from build123d import *

# Parameters (mm, degrees)
SKETCH1_W                      = 80
SKETCH1_H                      = 342
BOSS_EXTRUDE1_DEPTH            = 18
FILLET1_R                      = 50
CBORE_FOR_M5_SHCS1_D           = 5.5
CBORE_FOR_M5_SHCS1_DEPTH       = 28.347633298
CBORE_FOR_M5_SHCS1_CBORE_D     = 10
CBORE_FOR_M5_SHCS1_CBORE_DEPTH = 5
CBORE_FOR_M5_SHCS1_TIP         = 1.652366702
CHAMFER1_SIZE                  = 1
SKETCH5_R                      = 3.25
CUT_EXTRUDE1_DEPTH             = 284.418418597
CHAMFER2_SIZE                  = 1


with BuildPart() as part:
    # Sketch1 → Boss-Extrude1 (new body)
    with BuildSketch(Plane.XY):
        with Locations((41, 100)):
            Rectangle(SKETCH1_W, SKETCH1_H)
    extrude(amount=BOSS_EXTRUDE1_DEPTH)

    # Fillet1
    fillet1_edges = [part.edges().sort_by_distance(p)[0] for p in [
        (81, 271, 9),
        (81, -71, 9),
    ]]
    fillet(fillet1_edges, radius=FILLET1_R)

    # CBORE for M5 SHCS1
    with Locations(Plane.XY.offset(18)):
        with Locations((9.25, 250), (9.25, 190), (9.25, 130), (9.25, 70), (9.25, 10), (9.25, -50)):
            CounterBoreHole(CBORE_FOR_M5_SHCS1_D / 2, CBORE_FOR_M5_SHCS1_CBORE_D / 2, CBORE_FOR_M5_SHCS1_CBORE_DEPTH, depth=CBORE_FOR_M5_SHCS1_DEPTH)
            with Locations((0, 0, -(CBORE_FOR_M5_SHCS1_DEPTH + CBORE_FOR_M5_SHCS1_TIP / 2))):  # 118° drill point
                Cone(0, CBORE_FOR_M5_SHCS1_D / 2, CBORE_FOR_M5_SHCS1_TIP, mode=Mode.SUBTRACT)

    # Chamfer1
    chamfer1_edges = [part.edges().sort_by_distance(p)[0] for p in [
        (16, 271, 18),
        (81, 100, 18),
        (66.355339059, -56.355339059, 18),
        (66.355339059, 256.355339059, 18),
        (4.25, -50, 18),
        (4.25, 10, 18),
        (4.25, 70, 18),
        (1, 100, 18),
        (4.25, 130, 18),
        (4.25, 190, 18),
        (4.25, 250, 18),
        (16, -71, 18),
    ]]
    chamfer(chamfer1_edges, length=CHAMFER1_SIZE)

    # Sketch5 → Cut-Extrude1 (cut, through all)
    with BuildSketch(Plane.XY.offset(18)):
        with Locations((29.25, 40)):
            Circle(SKETCH5_R)
    extrude(amount=-CUT_EXTRUDE1_DEPTH, mode=Mode.SUBTRACT)

    # Chamfer2
    chamfer2_edges = [part.edges().sort_by_distance(p)[0] for p in [
        (26, 40, 0),
        (26, 40, 18),
    ]]
    chamfer(chamfer2_edges, length=CHAMFER2_SIZE)


solid = part.part
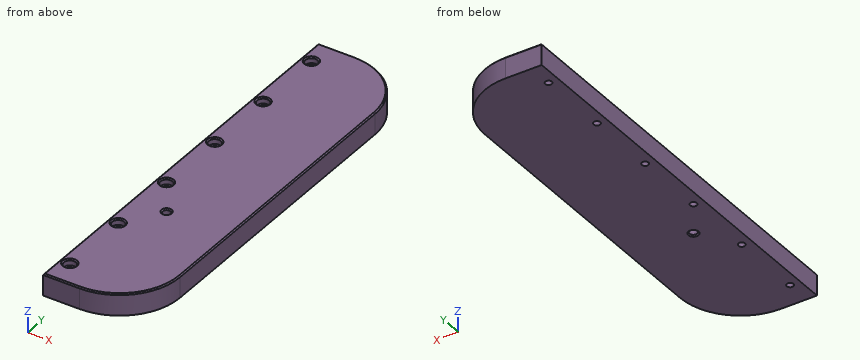
Source: CAD feature listing. Evaluate the final solid. Frame: model axes, mm. Round coordinates to 2 decimals unless told otherwise and drop trailing zeros. Write each loop counter-clockwise with the first axis right and the second up, starting at its lowest first coordinate (ties: lowest second). Pieces come first, ordered by that corner, then holes. Notation, with made-up numbers: M 51,36 L 79,36 A16 cw 79,49 Z; hole C 64,2 d4. An arc over 180 degrees is marked long. One line per item, written item: value. Start each with the question number.
Item 1: Section query A-A (z = 7.75). Return the cut outline in (x, y).
Item 2: Ray query, L1, parallel to X at y = 190, z = 3.75; L2, parallel to Y at x = 32, z = 12.5; L3, parallel to Z at x = 12.5, y = 11. Return the intervals inside material, ascending. Write a range as from..to.
Item 3: Pin query (flat end, axial travel): pin 1 (6.5 mm diameter, centred on x = 9.25, y = 70, fed in from +Z); pin 2 (1 mm diameter, centred on y = 232.5, z = 10, fed in from +X) (3 decimals); pin 3 (5 mm diameter, centred on x = 50.5, z = 13, fed in from +Y); pin 4 (5 mm diameter, centred on x = 9.25, y = 190, fed in from -Z). Return the tip coordinate at first contact, or that it passes through.
Result set:
1. outline: M 1,-71 L 31,-71 A50 ccw 81,-21 L 81,221 A50 ccw 31,271 L 1,271 Z; hole C 9.25,-50 d5.5; hole C 9.25,10 d5.5; hole C 9.25,70 d5.5; hole C 9.25,130 d5.5; hole C 9.25,190 d5.5; hole C 9.25,250 d5.5; hole C 29.25,40 d6.5
2. L1: x = 1..6.5, 12..81
2. L2: y = -70.99..38.27, 41.73..270.99
2. L3: z = 0..13
3. pin 1: stops at z = 13
3. pin 2: stops at x = 79.775
3. pin 3: stops at y = 268.02
3. pin 4: passes through
